For this review, use the dimensioned drawing (mm, ordinates from the lowest corner) and the shaded views. Coordinates: 2 decimals unless noted, no trailing zeros. Write each loop counter-clockwise with the first axis right and the second up, starting at its lowest first coordinate (ties: lowest second). Pieces come first, ordered by that corner, then holes. Notation, with made-up numbers: (85, 27.25) - (106, 27.25) arc R30 cw to (106, 50.25) - close; hole circle Ø1 at (3.25, 46.5). An arc over 180 degrees is marked (long way). Put each result on its own line as item: value.
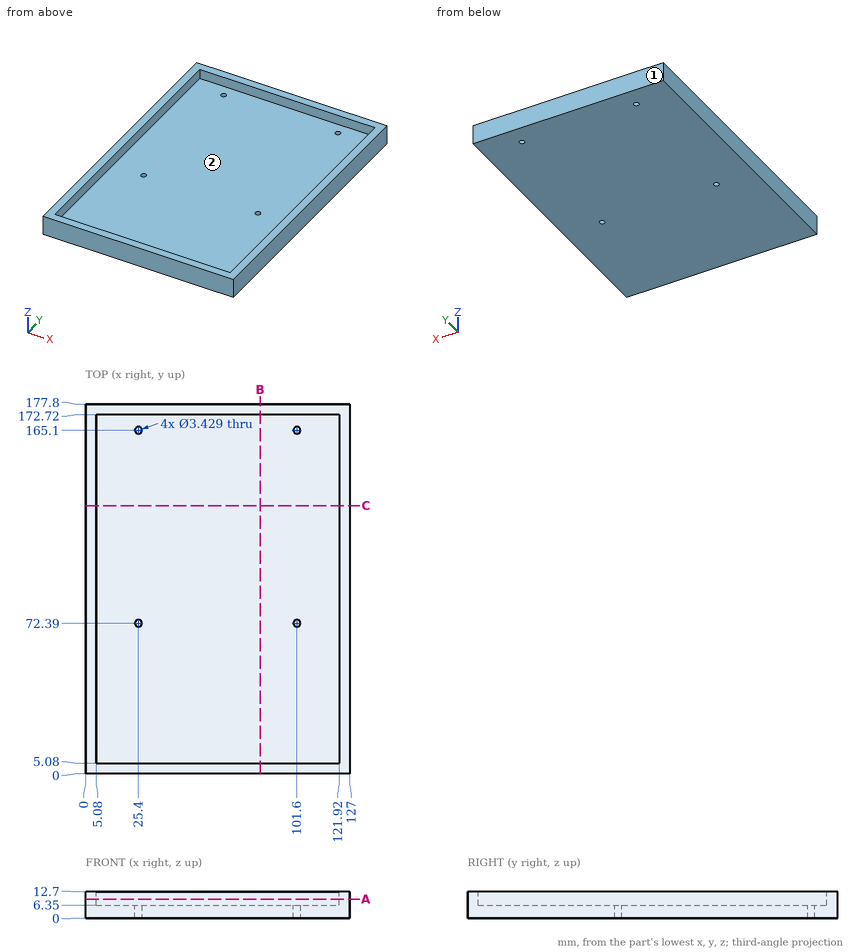
1. To check wall thickness, follow probe 1 along Y at (x, z) = (101.6, 2.5); probe 2 along X at (y, z) = (102, 9); probe 3 along X at (y, z) = (72.39, 5.25). State the ranges of each line that lie inside material, in increasing order.
Determined:
probe 1: y = 0 to 70.68, 74.1 to 163.39, 166.81 to 177.8
probe 2: x = 0 to 5.08, 121.92 to 127
probe 3: x = 0 to 23.69, 27.11 to 99.89, 103.31 to 127
2. Consider section A-A on z = 9.25. State the section outline as (x, y) points, plus the area to 3 significant figures.
Determined:
outline: (0, 0) - (127, 0) - (127, 177.8) - (0, 177.8) - close; hole (5.08, 5.08) - (121.92, 5.08) - (121.92, 172.72) - (5.08, 172.72) - close
area: 2,990 mm^2
3. The part is to be moulded in two halves that separate along X. For the marked faces 1 and 2, say which applies: +X half, -X half, draft (parallel to the pull), parting line (faces both ways), or undercut.
Determined:
face 1: draft
face 2: undercut
4. Consider section C-C on y = 129. State the section outline as (x, z) points.
Determined:
outline: (0, 0) - (127, 0) - (127, 12.7) - (121.92, 12.7) - (121.92, 6.35) - (5.08, 6.35) - (5.08, 12.7) - (0, 12.7) - close
5. Consider section B-B on x = 84. State the section outline as (y, z) points, plus the area to 3 significant figures.
Determined:
outline: (0, 0) - (177.8, 0) - (177.8, 12.7) - (172.72, 12.7) - (172.72, 6.35) - (5.08, 6.35) - (5.08, 12.7) - (0, 12.7) - close
area: 1,190 mm^2
6. For pin 1 Ø2 at (x, y) = (25.4, 165.1) entering from +Z (3 decimals); pin 2 Ø5.5 at (x, y) = (25.4, 72.39) entering from +Z, all flat-tipped, find the tip position at first contact; note any pin that passes through.
Determined:
pin 1: passes through
pin 2: stops at z = 6.35
